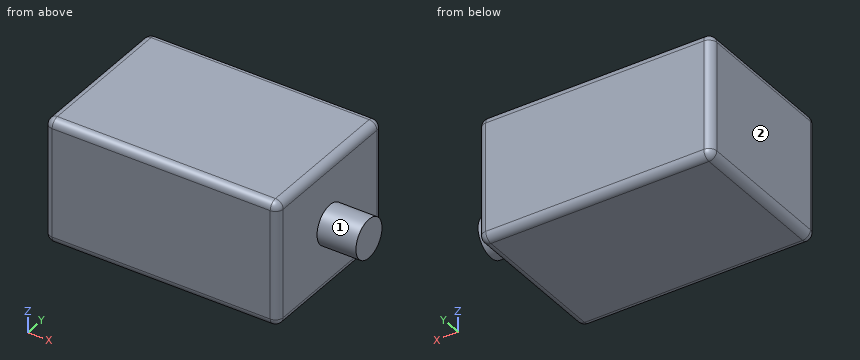
from build123d import *

# Parameters (mm, degrees)
SKETCH_1_W      = 30
SKETCH_1_H      = 20
EXTRUDE_1_DEPTH = 16
SKETCH_2_R      = 2.5
EXTRUDE_2_DEPTH = 5
FILLET_1_R      = 1


with BuildPart() as part:
    # 草图1 → 凸台-拉伸1 (new body)
    with BuildSketch(Plane.XY):
        Rectangle(SKETCH_1_W, SKETCH_1_H)
    extrude(amount=EXTRUDE_1_DEPTH)

    # 草图2 → 凸台-拉伸2 (add)
    with BuildSketch(Plane(origin=(15, 0, 0), x_dir=(0, 0, -1), z_dir=(1, 0, 0))):
        with Locations(Location((-8, 0, 0), (0, 0, 90))):
            Circle(SKETCH_2_R)
    extrude(amount=EXTRUDE_2_DEPTH)

    # 圆角1
    fillet_1_edges = [part.edges().sort_by_distance(p)[0] for p in [
        (-15, 0, 16),
        (0, -10, 16),
        (15, 0, 16),
        (0, -10, 0),
        (-15, 0, 0),
        (0, 10, 0),
        (15, 0, 0),
        (0, 10, 16),
        (15, -10, 8),
        (-15, -10, 8),
        (-15, 10, 8),
        (15, 10, 8),
    ]]
    fillet(fillet_1_edges, radius=FILLET_1_R)


solid = part.part
Geometry check sheet. Reference: the model listing, model coordinates, mm. Face numbers are marked on the shaded views. A direction names the side the tool comes from. Give positions to 0.01 mm unless a question says otherwise; leave off trailing zeros. Order: outer loops, then holes, each group sorted by start corner. A loop starts at its lowest first (then second) coordinate and runs counter-clockwise, first axis right, second up. Notation, with made-up numbers: M 77,23 L 122,23 A35 cw 122,57 Z; hole C -35,30.5 d11. An arc over 180 degrees is marked long. Use a Markdown table: item, result.
Item 1: Section check B-B (y = 1.5). Record the cut outline in (x, z).
Answers follow:
| item | result |
|---|---|
| outline | M -15,1 A1 ccw -14,0 L 14,0 A1 ccw 15,1 L 15,6 L 20,6 L 20,10 L 15,10 L 15,15 A1 ccw 14,16 L -14,16 A1 ccw -15,15 Z |
Item 2: Section check C-C (z = 4.5). Record the cut outline in (x, y).
Answers follow:
| item | result |
|---|---|
| outline | M -15,-9 A1 ccw -14,-10 L 14,-10 A1 ccw 15,-9 L 15,9 A1 ccw 14,10 L -14,10 A1 ccw -15,9 Z |
Item 3: Section check D-D (x = 16). Record the cut outline in (y, z), and give its area (3 significant figures).
Answers follow:
| item | result |
|---|---|
| outline | C 0,8 d5 |
| area | 19.6 mm2 |
Item 4: Depth check by flat-ended pin: P1, Ø1.5, axis at y = -5, z = 9.5, coming from the +X side. Enter the tip coordinate at first touch or a pass-through.
Answers follow:
| item | result |
|---|---|
| P1 | stops at x = 15 |
Item 5: Tool access check on the marked faces 1 and 2. Record the directions out of +Z, -Z, +X, -X, +Y, -Y that give a thin tool (end or side, any length) a straight path to the whole face; none if there is none.
Answers follow:
| item | result |
|---|---|
| face 1 | +X |
| face 2 | +Z, -Z, -X, +Y, -Y |
Item 6: Section check A-A (z = 8). Record the cut outline in (x, y), and give its area (3 significant figures).
Answers follow:
| item | result |
|---|---|
| outline | M -15,-9 A1 ccw -14,-10 L 14,-10 A1 ccw 15,-9 L 15,-2.5 L 20,-2.5 L 20,2.5 L 15,2.5 L 15,9 A1 ccw 14,10 L -14,10 A1 ccw -15,9 Z |
| area | 624 mm2 |
Item 7: Material ranges on line 1 along X through (y, z) = (4, 1.75), recorded low to high.
Answers follow:
| item | result |
|---|---|
| line 1 | x = -15 to 15 |
